Can you work these out from the model? Positions are in its coordinate system, mm. Round coordinates to 2 decimals unless told otherwise and drop trailing zeros. Loops run counter-clockwise (first coordinate to the right, second up) from the corner with the lowest first, then second, coordinate; pieces in that order, holes last.
(1) I want a section at B-B on x = 34. Write out the boundary of the cut face in (y, z).
(2) I want a section at A-A on z = 1.25. Give the number of separate pieces and of enclosed holes in the cut face, plus the area to 3 significant figures.
(3) I want a section at C-C on y = 42. Write out the boundary of the cut face in (x, z), plus the area to 3 significant figures.
(4) If I drill on line 1 along Y through (x, z) = (-1, 1.4); line 2 along Z through (x, y) = (14, -24.5), over which ranges is the centre line in solid material (lowest first)?
(5) Will this pin go through, and if not, where does the flat tip stop? pin 1 Ø8 at (x, y) = (-36, -32.5) entering from +Z.
from build123d import *

# Parameters (mm, degrees)
SKETCH_1_W      = 145
SKETCH_1_H      = 130
EXTRUDE_1_DEPTH = 1
SKETCH_2_W      = 2.25
SKETCH_2_H      = 2.15
EXTRUDE_2_DEPTH = 0.5


with BuildPart() as part:
    # 草图1 → 凸台-拉伸1 (new body)
    with BuildSketch(Plane.XY):
        Rectangle(SKETCH_1_W, SKETCH_1_H)
    extrude(amount=EXTRUDE_1_DEPTH)

    # 草图2 → 凸台-拉伸2 (add)
    with BuildSketch(Plane.XY.offset(1)):
        with Locations((-28.58, 51.063510548)):
            Rectangle(SKETCH_2_W, SKETCH_2_H)
        with Locations((-57.16, 51.063510548)):
            Rectangle(SKETCH_2_W, SKETCH_2_H)
        with Locations((0, 51.063510548)):
            Rectangle(SKETCH_2_W, SKETCH_2_H)
        with Locations((28.58, 51.063510548)):
            Rectangle(SKETCH_2_W, SKETCH_2_H)
        with Locations((57.16, 51.063510548)):
            Rectangle(SKETCH_2_W, SKETCH_2_H)
        with Locations((-28.58, 25.463510548)):
            Rectangle(SKETCH_2_W, SKETCH_2_H)
        with Locations((0, 25.463510548)):
            Rectangle(SKETCH_2_W, SKETCH_2_H)
        with Locations((28.58, 25.463510548)):
            Rectangle(SKETCH_2_W, SKETCH_2_H)
        with Locations((57.16, 25.463510548)):
            Rectangle(SKETCH_2_W, SKETCH_2_H)
        with Locations((-28.58, -0.136489452)):
            Rectangle(SKETCH_2_W, SKETCH_2_H)
        with Locations((0, -0.136489452)):
            Rectangle(SKETCH_2_W, SKETCH_2_H)
        with Locations((28.58, -0.136489452)):
            Rectangle(SKETCH_2_W, SKETCH_2_H)
        with Locations((57.16, -0.136489452)):
            Rectangle(SKETCH_2_W, SKETCH_2_H)
        with Locations((-28.58, -25.736489452)):
            Rectangle(SKETCH_2_W, SKETCH_2_H)
        with Locations((0, -25.736489452)):
            Rectangle(SKETCH_2_W, SKETCH_2_H)
        with Locations((28.58, -25.736489452)):
            Rectangle(SKETCH_2_W, SKETCH_2_H)
        with Locations((57.16, -25.736489452)):
            Rectangle(SKETCH_2_W, SKETCH_2_H)
        with Locations((-28.58, -51.336489452)):
            Rectangle(SKETCH_2_W, SKETCH_2_H)
        with Locations((0, -51.336489452)):
            Rectangle(SKETCH_2_W, SKETCH_2_H)
        with Locations((28.58, -51.336489452)):
            Rectangle(SKETCH_2_W, SKETCH_2_H)
        with Locations((57.16, -51.336489452)):
            Rectangle(SKETCH_2_W, SKETCH_2_H)
        with Locations((-57.16, 25.463510548)):
            Rectangle(SKETCH_2_W, SKETCH_2_H)
        with Locations((-57.16, -0.136489452)):
            Rectangle(SKETCH_2_W, SKETCH_2_H)
        with Locations((-57.16, -25.736489452)):
            Rectangle(SKETCH_2_W, SKETCH_2_H)
        with Locations((-57.16, -51.336489452)):
            Rectangle(SKETCH_2_W, SKETCH_2_H)
    extrude(amount=EXTRUDE_2_DEPTH)


solid = part.part
Filled sheet:
1. outline: (-65, 0) - (65, 0) - (65, 1) - (-65, 1) - close
2. separate pieces: 25
2. enclosed holes: 0
2. area: 121 mm2
3. outline: (-72.5, 0) - (72.5, 0) - (72.5, 1) - (-72.5, 1) - close
3. area: 145 mm2
4. line 1: y = -52.41 to -50.26, -26.81 to -24.66, -1.21 to 0.94, 24.39 to 26.54, 49.99 to 52.14
4. line 2: z = 0 to 1
5. pin 1: stops at z = 1
